```python
from build123d import *

# Parameters (mm, degrees)
BOSS_EXTRUDE2_DEPTH       = 5
SKETCH3_R                 = 1.0922
CUT_EXTRUDE2_DEPTH        = 2.2625
MIRROR27_START            = 3.5922
MIRROR27_DEPTH            = 1.4078
MIRROR27_2_DEPTH          = 1.4077999
MIRROR27_START_2          = 1.4077999
MIRROR27_3_DEPTH          = 2.1844001
MIRROR27_START_3          = -93
MIRROR27_4_OUTLINE_R      = 1.0922
MIRROR27_4_DEPTH          = 2.2625
TAP_DRILL_FOR_2_56_TAP1_D = 1.778


with BuildPart() as part:
    # Sketch1 → Boss-Extrude2 (new body)
    with BuildSketch(Plane(origin=(0, 0, 0), x_dir=(0, 0, -1), z_dir=(1, 0, 0))):
        with BuildLine():
            Line((2, 25), (7, 25))
            Line((7, 25), (7, 15.3375))
            ThreePointArc((7, 15.3375), (7.464967985, 14.214967985), (8.5875, 13.75))
            Line((8.5875, 13.75), (12.5, 13.75))
            ThreePointArc((12.5, 13.75), (15.151650429, 12.651650429), (16.25, 10))
            Line((16.25, 10), (16.25, 8.5875))
            ThreePointArc((16.25, 8.5875), (16.714967985, 7.464967985), (17.8375, 7))
            Line((17.8375, 7), (50, 7))
            Line((50, 7), (50, 2))
            Line((50, 2), (7, 2))
            Line((7, 2), (7, 7))
            Line((7, 7), (2, 7))
            Line((2, 7), (2, 25))
        make_face()
    boss_extrude2 = extrude(amount=BOSS_EXTRUDE2_DEPTH)

    # Sketch3 → Cut-Extrude2 (cut)
    with BuildSketch(Plane.XY.offset(-7)):
        with Locations((2.5, 4.5)):
            Circle(SKETCH3_R)
    cut_extrude2 = extrude(amount=-CUT_EXTRUDE2_DEPTH, mode=Mode.SUBTRACT)

    # Mirror26: Boss-Extrude2, Cut-Extrude2 across plane
    add(boss_extrude2.mirror(Plane.ZX.offset(25)))
    add(cut_extrude2.mirror(Plane.ZX.offset(25)), mode=Mode.SUBTRACT)

    # Mirror27: read off the stored shape, not the designer's step
    # Mirror27 outline → Mirror27 (add)
    with BuildSketch(Plane.YZ.offset(MIRROR27_START)):
        with BuildLine():
            ThreePointArc((15.3375, -93), (14.214967985, -92.535032015), (13.75, -91.4125))
            Line((13.75, -91.4125), (13.75, -87.5))
            ThreePointArc((13.75, -87.5), (12.651650429, -84.848349571), (10, -83.75))
            Line((10, -83.75), (8.5875, -83.75))
            ThreePointArc((8.5875, -83.75), (7.464967985, -83.285032015), (7, -82.1625))
            Line((7, -82.1625), (7, -50))
            Line((7, -50), (2, -50))
            Line((2, -50), (2, -93))
            Line((2, -93), (7, -93))
            Line((7, -93), (7, -98))
            Line((7, -98), (43, -98))
            Line((43, -98), (43, -93))
            Line((43, -93), (48, -93))
            Line((48, -93), (48, -50))
            Line((48, -50), (43, -50))
            Line((43, -50), (43, -82.1625))
            ThreePointArc((43, -82.1625), (42.535032015, -83.285032015), (41.4125, -83.75))
            Line((41.4125, -83.75), (40, -83.75))
            ThreePointArc((40, -83.75), (37.348349571, -84.848349571), (36.25, -87.5))
            Line((36.25, -87.5), (36.25, -91.4125))
            ThreePointArc((36.25, -91.4125), (35.785032015, -92.535032015), (34.6625, -93))
            Line((34.6625, -93), (15.3375, -93))
        make_face()
    extrude(amount=MIRROR27_DEPTH)

    # Mirror27 2 outline → Mirror27 2 (add)
    with BuildSketch(Plane.YZ):
        with BuildLine():
            ThreePointArc((15.3375, -93), (14.214967985, -92.535032015), (13.75, -91.4125))
            Line((13.75, -91.4125), (13.75, -87.5))
            ThreePointArc((13.75, -87.5), (12.651650429, -84.848349571), (10, -83.75))
            Line((10, -83.75), (8.5875, -83.75))
            ThreePointArc((8.5875, -83.75), (7.464967985, -83.285032015), (7, -82.1625))
            Line((7, -82.1625), (7, -50))
            Line((7, -50), (2, -50))
            Line((2, -50), (2, -93))
            Line((2, -93), (7, -93))
            Line((7, -93), (7, -98))
            Line((7, -98), (43, -98))
            Line((43, -98), (43, -93))
            Line((43, -93), (48, -93))
            Line((48, -93), (48, -50))
            Line((48, -50), (43, -50))
            Line((43, -50), (43, -82.1625))
            ThreePointArc((43, -82.1625), (42.535032015, -83.285032015), (41.4125, -83.75))
            Line((41.4125, -83.75), (40, -83.75))
            ThreePointArc((40, -83.75), (37.348349571, -84.848349571), (36.25, -87.5))
            Line((36.25, -87.5), (36.25, -91.4125))
            ThreePointArc((36.25, -91.4125), (35.785032015, -92.535032015), (34.6625, -93))
            Line((34.6625, -93), (15.3375, -93))
        make_face()
    extrude(amount=MIRROR27_2_DEPTH)

    # Mirror27 3 outline → Mirror27 3 (add)
    with BuildSketch(Plane.YZ.offset(MIRROR27_START_2)):
        with BuildLine():
            ThreePointArc((15.3375, -93), (14.214967985, -92.535032015), (13.75, -91.4125))
            Line((13.75, -91.4125), (13.75, -87.5))
            ThreePointArc((13.75, -87.5), (12.651650429, -84.848349571), (10, -83.75))
            Line((10, -83.75), (8.5875, -83.75))
            ThreePointArc((8.5875, -83.75), (7.464967985, -83.285032015), (7, -82.1625))
            Line((7, -82.1625), (7, -50))
            Line((7, -50), (2, -50))
            Line((2, -50), (2, -93))
            Line((2, -93), (7, -93))
            Line((7, -93), (7, -98))
            Line((7, -98), (43, -98))
            Line((43, -98), (43, -93))
            Line((43, -93), (48, -93))
            Line((48, -93), (48, -50))
            Line((48, -50), (43, -50))
            Line((43, -50), (43, -82.1625))
            ThreePointArc((43, -82.1625), (42.535032015, -83.285032015), (41.4125, -83.75))
            Line((41.4125, -83.75), (40, -83.75))
            ThreePointArc((40, -83.75), (37.348349571, -84.848349571), (36.25, -87.5))
            Line((36.25, -87.5), (36.25, -91.4125))
            ThreePointArc((36.25, -91.4125), (35.785032015, -92.535032015), (34.6625, -93))
            Line((34.6625, -93), (15.3375, -93))
        make_face()
    extrude(amount=MIRROR27_3_DEPTH)

    # Mirror27 4 outline → Mirror27 4 (cut)
    with BuildSketch(Plane.XY.offset(MIRROR27_START_3)):
        with Locations((2.5, 4.5)):
            Circle(MIRROR27_4_OUTLINE_R)
        with Locations((2.5, 45.5)):
            Circle(MIRROR27_4_OUTLINE_R)
    extrude(amount=MIRROR27_4_DEPTH, mode=Mode.SUBTRACT)

    # Tap Drill for #2-56 Tap1 (through all)
    with Locations(Plane.ZY):
        with Locations((-87.5, 10), (-87.5, 40), (-12.5, 40), (-12.5, 10)):
            Hole(TAP_DRILL_FOR_2_56_TAP1_D / 2)


solid = part.part
```
Work out the finished part from the listing and answer in its coordinate system (mm). A direction names the side the tool comes from. Coordinates: 2 decimals unless noted, no trailing zeros. Write each loop counter-clockwise with the first axis right and the second up, starting at its lowest first coordinate (ties: lowest second). Pieces come first, ordered by that corner, then holes. Notation, with made-up numbers: (48, 10) - (93, 10) arc R14 ccw to (93, 16) - close; hole circle Ø11 at (-20, 10.25). An arc over 180 degrees is marked (long way). Answer as a JSON object with one key per item and string values.
Q1. Find section C-C (y = 4.5). Write down the section's boundary in (x, z), plus the area to 3 significant figures.
Results list:
{"outline": "(0, -93) - (1.41, -93) - (1.41, -90.74) - (3.59, -90.74) - (3.59, -93) - (5, -93) - (5, -7) - (3.59, -7) - (3.59, -9.26) - (1.41, -9.26) - (1.41, -7) - (0, -7) - close", "area": "420 mm^2"}
Q2. Consider L1, parallel to Z at x = 3.4, y = 40; L2, parallel to Y at x = 3, z = -79.5; L3, parallel to Y at x = 3.7, z = -12.5. Determine where each line is inside the solid, lowest interval first. Write a range as from..to.
Results list:
{"L1": "z = -98..-88.39, -86.61..-83.75, -16.25..-13.39, -11.61..-2", "L2": "y = 2..7, 43..48", "L3": "y = 2..9.11, 10.89..13.75, 36.25..39.11, 40.89..48"}
Q3. For a pull along X with two mould halves and no side action, classify faces 1 (the flat face through (5, 6, -53)), 2 (the flat face through (2, 25, -2)), 3 (the flat face through (2, 46, -90.738)) as pulls with the +X half, pulls with the -X half, needs draft (parallel to the pull), parting line crosses it, or undercut.
Results list:
{"face 1": "pulls with the +X half", "face 2": "needs draft", "face 3": "undercut"}
Q4. Find section A-A (y = 27.5). Write down the section's boundary in (x, z), plus the area to 3 significant figures.
Results list:
{"outline": "(0, -98) - (5, -98) - (5, -93) - (0, -93) - close; (0, -7) - (5, -7) - (5, -2) - (0, -2) - close", "area": "50.0 mm^2"}
Q5. Which of the six approach directions +Z, -Z, +X, -X, +Y, -Y give full straight-line access (tool end or side, diameter ignored) to faces 4 (the flat face through (2, 7, -95)), 5 (the cylindrical face through (2.5, 12.7, -15.1)), 6 (the flat face through (2, 43, -5))?
Results list:
{"face 4": "-Z, +X, -X, -Y", "face 5": "+X, -X", "face 6": "+Z, +X, -X, +Y"}
Q6. Given pin 1 Ø1.7 at (x, y) = (2.5, 4.5) entering from +Z; pin 2 Ø1.5 at (x, z) = (2, -95.5) entering from +Y; pin 3 Ø1.6 at (y, z) = (10, -87.5) entering from +X; pin 4 Ø2.5 at (x, y) = (3.5, 5.5) entering from -Z, each flat-ended and moving along its own axis, determine where each tip first touches the part or whether it passes through.
Results list:
{"pin 1": "stops at z = -9.26", "pin 2": "stops at y = 43", "pin 3": "passes through", "pin 4": "stops at z = -93"}
Q7. Find section B-B (z = -79.5). Write down the section's boundary in (x, y), plus the area to 3 significant figures.
Results list:
{"outline": "(0, 2) - (5, 2) - (5, 7) - (0, 7) - close; (0, 43) - (5, 43) - (5, 48) - (0, 48) - close", "area": "50.0 mm^2"}
